```python
from build123d import *

# Parameters (mm, degrees)
F1_DEPTH = 25
F2_W     = 1.9
F2_H     = 1
F2_W_2   = 10.6
F3_DEPTH = 9
F4_SIZE  = 0.6


with BuildPart() as f1:
    # F0 (on Front) → F1 (new body, symmetric)
    with BuildSketch(Plane.XZ):
        Polygon((-9.35, -6), (9.35, -6), (9.35, 6), (4.35, 6), (4.35, -2), (-4.35, -2), (-4.35, 6), (-9.35, 6), align=None)
    extrude(amount=F1_DEPTH, both=True)

    # F2 (on face) → F3 (cut)
    with BuildSketch(Plane.XY.offset(6)):
        with Locations((5.3, 0)):
            Rectangle(F2_W, F2_H)
        with Locations((-0.95, 0)):
            Rectangle(F2_W_2, F2_H)
    extrude(amount=-F3_DEPTH, mode=Mode.SUBTRACT)

    # F4 (call 1 of 10: OpenCascade refuses the feature's edges together)
    f4_edges = [f1.edges().sort_by_distance(p)[0] for p in [
        (5.3, 0.5, 6),
        (6.25, 0, 6),
        (5.3, -0.5, 6),
        (4.35, 12.75, 6),
        (4.35, -12.75, 6),
    ]]
    chamfer(f4_edges, length=F4_SIZE)

    # F4#2 (call 2 of 10)
    f4_2_edges = [f1.edges().sort_by_distance(p)[0] for p in [
        (-5.3, 0.5, 6),
        (-6.25, 0, 6),
        (-5.3, -0.5, 6),
        (-4.35, -12.75, 6),
        (-4.35, 12.75, 6),
    ]]
    chamfer(f4_2_edges, length=F4_SIZE)

    # F4#3 (call 3 of 10)
    f4_3_edges = [f1.edges().sort_by_distance(p)[0] for p in [
        (9.35, 0, 6),
    ]]
    chamfer(f4_3_edges, length=F4_SIZE)

    # F4#4 (call 4 of 10)
    f4_4_edges = [f1.edges().sort_by_distance(p)[0] for p in [
        (-9.35, 0, 6),
    ]]
    chamfer(f4_4_edges, length=F4_SIZE)

    # F4#5 (call 5 of 10)
    f4_5_edges = [f1.edges().sort_by_distance(p)[0] for p in [
        (0, 25, -6),
    ]]
    chamfer(f4_5_edges, length=F4_SIZE)

    # F4#6 (call 6 of 10)
    f4_6_edges = [f1.edges().sort_by_distance(p)[0] for p in [
        (0, -25, -6),
    ]]
    chamfer(f4_6_edges, length=F4_SIZE)

    # F4#7 (call 7 of 10)
    f4_7_edges = [f1.edges().sort_by_distance(p)[0] for p in [
        (-6.25, 0, -3),
    ]]
    chamfer(f4_7_edges, length=F4_SIZE)

    # F4#8 (call 8 of 10)
    f4_8_edges = [f1.edges().sort_by_distance(p)[0] for p in [
        (6.25, 0, -3),
    ]]
    chamfer(f4_8_edges, length=F4_SIZE)

    # F4#9 (call 9 of 10)
    f4_9_edges = [f1.edges().sort_by_distance(p)[0] for p in [
        (0, 0.5, -2),
    ]]
    chamfer(f4_9_edges, length=F4_SIZE)

    # F4#10 (call 10 of 10)
    f4_10_edges = [f1.edges().sort_by_distance(p)[0] for p in [
        (0, -0.5, -2),
    ]]
    chamfer(f4_10_edges, length=F4_SIZE)


solid = f1.part
```
Design review of the part built by this model. Coordinates are the model's own, in mm. A direction names the side the tool comes from. Coordinates: 2 decimals unless noted, no trailing zeros. Loops run counter-clockwise (first coordinate to the right, second up) from the corner with the lowest first, then second, coordinate; pieces in that order, holes last. Notation, with made-up numbers: M 47,54 L 92,54 A8 ccw 92,59 Z; hole C 57,-40 d5. An arc over 180 degrees is marked long. One line per question, with ' | ' between items.
(1) We need section C-C (x = 1.75). Give the boundary of the cut face in (y, z), and give its area (3 significant figures).
Filled in:
outline: M -25,-5.4 L -24.4,-6 L 24.4,-6 L 25,-5.4 L 25,-2 L 1.1,-2 L 0.5,-2.6 L 0.5,-3 L -0.5,-3 L -0.5,-2.6 L -1.1,-2 L -25,-2 Z | area: 198 mm^2
(2) For pin 1 Ø0.8 at (x, y) = (2, 0) entering from +Z; pin 2 Ø2 at (x, y) = (-2.5, 17.5) entering from +Z, all flat-tipped, find the tip position at first contact; note any pin that passes through.
Filled in:
pin 1: stops at z = -3 | pin 2: stops at z = -2
(3) Machinability: for faces 4 (the face through (9.35, 0, 0)), 5 (the face through (0, 0, -3)), 6 (the face through (4.35, -13, 1)), which of the approach directions +Z, -Z, +X, -X, +Y, -Y give a long, thin tool a straight path to every point of the face, cutting with its end or side? Answer none if there is none.
Filled in:
face 4: +Z, -Z, +X, +Y, -Y | face 5: +Z | face 6: +Z, +Y, -Y
(4) We need section A-A (z = 1.5). Give the boundary of the cut face in (x, y), and give its area (3 significant figures).
Filled in:
outline: M -9.35,-25 L -4.35,-25 L -4.35,-0.5 L -6.25,-0.5 L -6.25,0.5 L -4.35,0.5 L -4.35,25 L -9.35,25 Z; M 4.35,-25 L 9.35,-25 L 9.35,25 L 4.35,25 L 4.35,0.5 L 6.25,0.5 L 6.25,-0.5 L 4.35,-0.5 Z | area: 496 mm^2
(5) Draft analysis for pull direction Y (two halves, no side actions). For faces 1 (the face through (-0.1, -25, -2.2)), 2 (the face through (-9.35, 0, 0)), 3 (the face through (6.25, 0, 2)), state which applies: released by +Y, released by -Y, zero draft, split by the parting line, or undercut.
Filled in:
face 1: released by -Y | face 2: zero draft | face 3: undercut
(6) Wall thickness on probe 1 along X at (y, z) = (4.5, 4.75); probe 2 along Z at (x, y) = (1.75, 4); probe 3 along Y at (x, z) = (-0.5, -2.25): over which ranges is each line inside the solid? List them lowest first.
Filled in:
probe 1: x = -9.35 to -4.35, 4.35 to 9.35 | probe 2: z = -6 to -2 | probe 3: y = -25 to -0.85, 0.85 to 25
(7) We need section B-B (y = 10). Give the boundary of the cut face in (x, z), and give its area (3 significant figures).
Filled in:
outline: M -9.35,-6 L 9.35,-6 L 9.35,5.4 L 8.75,6 L 4.95,6 L 4.35,5.4 L 4.35,-2 L -4.35,-2 L -4.35,5.4 L -4.95,6 L -8.75,6 L -9.35,5.4 Z | area: 154 mm^2
(8) We need section D-D (y = 0). Give the boundary of the cut face in (x, z), and give its area (3 significant figures).
Filled in:
outline: M -9.35,-6 L 9.35,-6 L 9.35,5.4 L 8.75,6 L 6.85,6 L 6.25,5.4 L 6.25,-2.4 L 5.65,-3 L -5.65,-3 L -6.25,-2.4 L -6.25,5.4 L -6.85,6 L -8.75,6 L -9.35,5.4 Z | area: 112 mm^2
